```python
from build123d import *

# Parameters (mm, degrees)
SKETCH2_R                       = 25
BOSS_EXTRUDE1_DEPTH             = 5.5
CHAMFER1_SIZE                   = 1
CHAMFER1_SIZE2                  = 0.577350269
SKETCH3_R                       = 7
BOSS_EXTRUDE2_DEPTH             = 2.5
M3X0_5_TAPPED_HOLE1_D           = 2.5
M3X0_5_TAPPED_HOLE1_CSINK_D     = 3.25
M3X0_5_TAPPED_HOLE1_CSINK_ANGLE = 60
SKETCH8_R                       = 4
CUT_EXTRUDE1_DEPTH              = 37.249137921
CUT_EXTRUDE2_DEPTH              = 36.780581326
CUT_EXTRUDE3_DEPTH              = 36.780581326
CIRPATTERN1_COUNT               = 4
BOSS_EXTRUDE3_START             = 2.5
SKETCH11_R                      = 25
SKETCH11_R_2                    = 21.5
BOSS_EXTRUDE3_DEPTH             = 2.5


with BuildPart() as part:
    # Sketch2 → Boss-Extrude1 (new body)
    with BuildSketch(Plane(origin=(0, 0, 0), x_dir=(1, 0, 0), z_dir=(0, 1, 0))):
        with Locations(Location((0, 0, 0), (0, 0, 270))):
            Circle(SKETCH2_R)
    extrude(amount=BOSS_EXTRUDE1_DEPTH)

    # Chamfer1
    chamfer1_edges = [part.edges().sort_by_distance(p)[0] for p in [
        (0, 5.5, -25),
    ]]
    chamfer1_side = [part.faces().sort_by_distance(p)[0] for p in [
        (0, 2.75, -25),
    ]]
    chamfer(chamfer1_edges, length=CHAMFER1_SIZE, length2=CHAMFER1_SIZE2, reference=chamfer1_side[0])

    # Sketch3 → Boss-Extrude2 (add)
    with BuildSketch(Plane(origin=(0, 5.5, 0), x_dir=(1, 0, 0), z_dir=(0, 1, 0))):
        with Locations(Location((0, 0, 0), (0, 0, 270))):
            Circle(SKETCH3_R)
    extrude(amount=BOSS_EXTRUDE2_DEPTH)

    # M3x0.5 Tapped Hole1 (through all)
    with Locations(Plane(origin=(0, 5.5, 0), x_dir=(1, 0, 0), z_dir=(0, 1, 0))):
        with Locations((0, 10)):
            m3x0_5_tapped_hole1 = CounterSinkHole(M3X0_5_TAPPED_HOLE1_D / 2, M3X0_5_TAPPED_HOLE1_CSINK_D / 2, counter_sink_angle=M3X0_5_TAPPED_HOLE1_CSINK_ANGLE)

    # Sketch8 → Cut-Extrude1 (cut, through all)
    with BuildSketch(Plane(origin=(0, 8, 0), x_dir=(1, 0, 0), z_dir=(0, 1, 0))):
        with Locations(Location((0, 0, 0), (0, 0, 270))):
            Circle(SKETCH8_R)
    extrude(amount=-CUT_EXTRUDE1_DEPTH, mode=Mode.SUBTRACT)

    # Sketch9 → Cut-Extrude2 (cut, through all)
    with BuildSketch(Plane(origin=(0, 5.5, 0), x_dir=(1, 0, 0), z_dir=(0, 1, 0))):
        with BuildLine():
            Line((4, 32.5), (4, 17.5))
            ThreePointArc((4, 17.5), (0, 13.5), (-4, 17.5))
            Line((-4, 17.5), (-4, 32.5))
            ThreePointArc((-4, 32.5), (0, 36.5), (4, 32.5))
        make_face()
    cut_extrude2 = extrude(amount=-CUT_EXTRUDE2_DEPTH, mode=Mode.SUBTRACT)

    # Sketch10 → Cut-Extrude3 (cut, through all)
    with BuildSketch(Plane(origin=(0, 5.5, 0), x_dir=(1, 0, 0), z_dir=(0, 1, 0))):
        with BuildLine():
            Line((-23.539452544, 29.196306793), (-5.342535685, 10.999389935))
            ThreePointArc((-5.342535685, 10.999389935), (-5.342535685, 5.342535685), (-10.999389935, 5.342535685))
            Line((-10.999389935, 5.342535685), (-29.196306793, 23.539452544))
            ThreePointArc((-29.196306793, 23.539452544), (-29.196306793, 29.196306793), (-23.539452544, 29.196306793))
        make_face()
    cut_extrude3 = extrude(amount=-CUT_EXTRUDE3_DEPTH, mode=Mode.SUBTRACT)

    # CirPattern1: M3x0.5 Tapped Hole1, Cut-Extrude2, Cut-Extrude3 ×4 about axis
    cirpattern1_axis = Axis((0, 0, 0), (0, 1, 0))
    add([m3x0_5_tapped_hole1.rotate(cirpattern1_axis, i * 360 / CIRPATTERN1_COUNT) for i in range(1, CIRPATTERN1_COUNT)], mode=Mode.SUBTRACT)
    add([cut_extrude2.rotate(cirpattern1_axis, i * 360 / CIRPATTERN1_COUNT) for i in range(1, CIRPATTERN1_COUNT)], mode=Mode.SUBTRACT)
    add([cut_extrude3.rotate(cirpattern1_axis, i * 360 / CIRPATTERN1_COUNT) for i in range(1, CIRPATTERN1_COUNT)], mode=Mode.SUBTRACT)

    # Sketch11 → Boss-Extrude3 (add)
    with BuildSketch(Plane.XZ.offset(BOSS_EXTRUDE3_START)):
        with Locations(Location((0, 0, 0), (0, 0, 270))):
            Circle(SKETCH11_R)
        with Locations(Location((0, 0, 0), (0, 0, 79.277847584))):
            Circle(SKETCH11_R_2, mode=Mode.SUBTRACT)
    extrude(amount=-BOSS_EXTRUDE3_DEPTH)


solid = part.part
```
Here's how the part is built. I have some questions about the finished solid (model axes, mm). A direction names the side the tool comes from. Round coordinates to 2 decimals unless told otherwise and drop trailing zeros. Write each loop counter-clockwise with the first axis right and the second up, starting at its lowest first coordinate (ties: lowest second). Pieces come first, ordered by that corner, then holes.
Q1. If we mould it in two halves opening along X, with no side actions, what happens to faces 1 (the flat face through (4, 3, -21)), 2 (the cylindrical face through (-9.58, 0.17, -23.09)), 3 (the flat face through (-4, 3, -21)), 4 (the conical face through (-9.357, 5.118, -22.798))? For each: +X half, -X half, draft (parallel to the pull), parting line (faces both ways), or undercut.
Q2. Which directions (+Z, -Z, +X, -X, +Y, -Y) give clear straight access to the entire face, cutting with the end or side of a thin tool? Please do faces 5 (the flat face through (-5, 5.5, -11)), 6 (the flat face through (0, 0, -5)), 7 (the flat face through (-4, 3, 21)), 8 (the flat face through (21, 3, -4)).
Q3. If we section it at C-C on z = -16: Write out the boundary of the cut face in (x, y), plus the area to 3 significant figures.
Q4. Will these pins go through, and if not, where does the flat tip stop? P1, Ø2, axis at x = 0, z = -10, coming from the -Y side; P2, Ø8, axis at x = -4.5, z = 13, coming from the +Y side; P3, Ø3, axis at y = 1, z = -9, coming from the +X side; P4, Ø3, axis at y = 2, z = -21.5, coming from the +X side.
Q5. If we section it at A-A on z = 0: Give the number of separate pieces and of enclosed holes in the cut face, plus the area to 3 significant figures.
Q6. Please list where these lines run through material, in increasing order: probe 1 along X at (y, z) = (2.05, 0); probe 2 along Z at (x, y) = (-10, 2.95); probe 3 along X at (y, z) = (1.75, -14).
Q7. If we section it at D-D on x = -16.5: Write out the boundary of the cut face in (y, z).
Answer below:
1. face 1: undercut
1. face 2: parting line
1. face 3: undercut
1. face 4: -X half
2. face 5: +Y
2. face 6: -Y
2. face 7: +Z, +Y
2. face 8: +X, +Y
3. outline: (-19.21, -2.5) - (-14.36, -2.5) - (-14.36, 0) - (-19.21, 0) - close; (-10.34, 0) - (-3.71, 0) - (-3.71, 5.5) - (-10.34, 5.5) - close; (3.71, 0) - (10.34, 0) - (10.34, 5.5) - (3.71, 5.5) - close; (14.36, -2.5) - (19.21, -2.5) - (19.21, 0) - (14.36, 0) - close
3. area: 97.2 mm2
4. P1: passes through
4. P2: stops at y = 5.5
4. P3: stops at x = 23.85
4. P4: stops at x = 14.62
5. separate pieces: 6
5. enclosed holes: 0
5. area: 109 mm2
6. probe 1: x = -13.5 to -11.25, -8.75 to -4, 4 to 8.75, 11.25 to 13.5
6. probe 2: z = -22.91 to -15.66, -4.61 to -1.25, 1.25 to 4.61, 15.66 to 22.91
6. probe 3: x = -20.71 to -19.66, -8.34 to -1.94, 1.94 to 8.34, 19.66 to 20.71
7. outline: (-2.5, -18.78) - (0, -18.78) - (0, -13.78) - (-2.5, -13.78) - close; (-2.5, 13.78) - (0, 13.78) - (0, 18.78) - (-2.5, 18.78) - close; (0, -10.84) - (5.5, -10.84) - (5.5, -3.87) - (0, -3.87) - close; (0, 3.87) - (5.5, 3.87) - (5.5, 10.84) - (0, 10.84) - close
